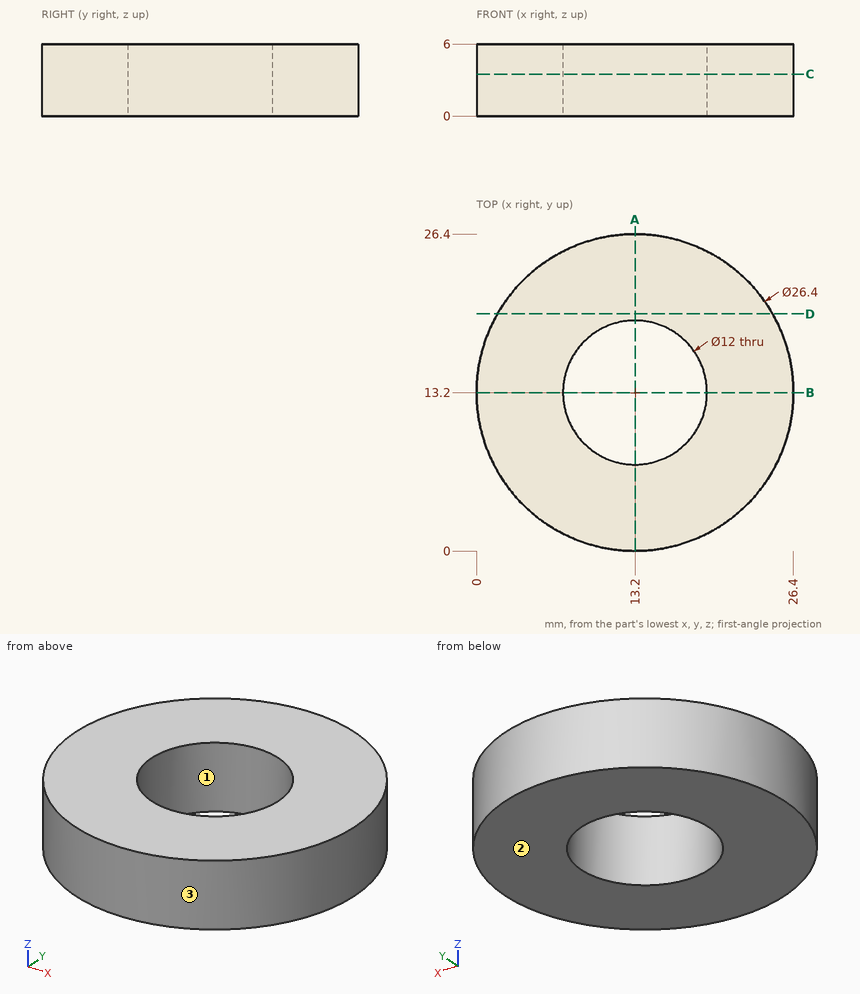
Check sheet for the drawn part. Datum: minimum x, y, z corner. Units: mm. Give positions to 0.01 mm unless a question says otherwise; leave off trailing zeros. Order: outer loops, then holes, each group sorted by start corner. A loop starts at its lowest first (then second) coordinate and runs counter-clockwise, first axis right, second up.
1. Scan lines: line 1 (Y direction, x = 13.2, z = 2.5); line 2 (Y direction, x = 10.25, z = 0.45); line 3 (X direction, y = 15.5, z = 2.05). Record each from-to range of solid material in increasing order.
Completed:
line 1: y = 0 to 7.2, 19.2 to 26.4
line 2: y = 0.33 to 7.98, 18.42 to 26.07
line 3: x = 0.2 to 7.66, 18.74 to 26.2
2. Sectioned sample at C-C (z = 3.5). Record the boundary of the cut face in (x, y), then the cut area to 3 significant figures.
Completed:
outline: circle Ø26.4 at (13.2, 13.2); hole circle Ø12 at (13.2, 13.2)
area: 434 mm2
3. Draft check along Y on the marked faces 1, 2 and 3. Enter one of: pulls with the +Y half, pulls with the -Y half, needs draft (parallel to the pull), parting line crosses it, or undercut.
Completed:
face 1: undercut
face 2: needs draft
face 3: parting line crosses it
4. Sectioned sample at A-A (x = 13.2). Record the boundary of the cut face in (y, z), then the cut area to 3 significant figures.
Completed:
outline: (0, 0) - (7.2, 0) - (7.2, 6) - (0, 6) - close; (19.2, 0) - (26.4, 0) - (26.4, 6) - (19.2, 6) - close
area: 86.4 mm2
5. Depth check by flat-ended pin: pin 1 (3 mm diameter, centred on x = 16, y = 6.5, fed in from -Z); pin 2 (11 mm diameter, centred on x = 13.2, y = 13.2, fed in from -Z). Enter the tip coordinate at first touch or a pass-through.
Completed:
pin 1: stops at z = 0
pin 2: passes through
6. Sectioned sample at D-D (y = 19.75). Record the boundary of the cut face in (x, z).
Completed:
outline: (1.74, 0) - (24.66, 0) - (24.66, 6) - (1.74, 6) - close
